For this review, take the finished solid that the model builds, in its own axes (mm). Give positions to 0.01 mm unless a question says otherwise; leave off trailing zeros. Order: outer loops, then holes, each group sorted by start corner. A loop starts at its lowest first (then second) coordinate and runs counter-clockwise, first axis right, second up. Notation, with made-up numbers: (43, -29.5) - (51, -29.5) arc R23 cw to (51, -8.5) - close; hole circle Ø11 at (88, 55.5). An arc over 180 degrees is marked (long way). One line per item, written item: value.
```python
from build123d import *

# Parameters (mm, degrees)
BOX032_W     = 40
BOX032_H     = 17
BOX032_DEPTH = 40
BOX033_W     = 40
BOX033_H     = 17
BOX033_DEPTH = 40
BOX029_W     = 330
BOX029_H     = 20
BOX029_DEPTH = 40
BOX030_W     = 30
BOX030_H     = 330
BOX030_DEPTH = 40
BOX031_W     = 30
BOX031_H     = 330
BOX031_DEPTH = 40
BOX028_W     = 330
BOX028_H     = 20
BOX028_DEPTH = 40
BOX009_W     = 64.5
BOX009_H     = 12
BOX009_DEPTH = 3
BOX008_W     = 64.5
BOX008_H     = 10
BOX008_DEPTH = 3
BOX007_W     = 22
BOX007_H     = 6
BOX007_DEPTH = 3
BOX006_W     = 22
BOX006_H     = 6
BOX006_DEPTH = 3
BOX005_W     = 22
BOX005_H     = 6
BOX005_DEPTH = 3
BOX004_W     = 74.5
BOX004_H     = 117
BOX004_DEPTH = 10
BOX003_W     = 74.5
BOX003_H     = 117
BOX003_DEPTH = 10
BOX002_W     = 74.5
BOX002_H     = 117
BOX002_DEPTH = 10
BOX_W        = 310
BOX_H        = 310
BOX_DEPTH    = 3
BOX010_W     = 64.5
BOX010_H     = 12
BOX010_DEPTH = 3


with BuildPart() as cube031:
    # Box032 → Box032 (new body)
    with BuildSketch(Plane(origin=(-20, 140, 0), x_dir=(1, 0, 0), z_dir=(0, 0, 1))):
        with Locations((20, 8.5)):
            Rectangle(BOX032_W, BOX032_H)
    extrude(amount=BOX032_DEPTH)


with BuildPart() as fusion001010002020:
    # Box033 → Box033 (new body)
    with BuildSketch(Plane(origin=(-20, -156, 0), x_dir=(1, 0, 0), z_dir=(0, 0, 1))):
        with Locations((20, 8.5)):
            Rectangle(BOX033_W, BOX033_H)
    extrude(amount=BOX033_DEPTH)

    # Fusion001010002020: union Cube031
    add(cube031.part)


with BuildPart() as cube028:
    # Box029 → Box029 (new body)
    with BuildSketch(Plane(origin=(-165, -159, 0), x_dir=(1, 0, 0), z_dir=(0, 0, 1))):
        with Locations((165, 10)):
            Rectangle(BOX029_W, BOX029_H)
    extrude(amount=BOX029_DEPTH)


with BuildPart() as cube029:
    # Box030 → Box030 (new body)
    with BuildSketch(Plane(origin=(-170, -170, 0), x_dir=(1, 0, 0), z_dir=(0, 0, 1))):
        with Locations((15, 165)):
            Rectangle(BOX030_W, BOX030_H)
    extrude(amount=BOX030_DEPTH)


with BuildPart() as cube030:
    # Box031 → Box031 (new body)
    with BuildSketch(Plane(origin=(140, -170, 0), x_dir=(1, 0, 0), z_dir=(0, 0, 1))):
        with Locations((15, 165)):
            Rectangle(BOX031_W, BOX031_H)
    extrude(amount=BOX031_DEPTH)


with BuildPart() as cut007:
    # Box028 → Box028 (new body)
    with BuildSketch(Plane(origin=(-165, 140, 0), x_dir=(1, 0, 0), z_dir=(0, 0, 1))):
        with Locations((165, 10)):
            Rectangle(BOX028_W, BOX028_H)
    extrude(amount=BOX028_DEPTH)

    # Fusion001010002021: union Cube028, Cube029, Cube030
    add(cube028.part)
    add(cube029.part)
    add(cube030.part)

    # Cut007: cut Fusion001010002020
    add(fusion001010002020.part, mode=Mode.SUBTRACT)


with BuildPart() as cube008:
    # Box009 → Box009 (new body)
    with BuildSketch(Plane(origin=(80.5, -72, 28), x_dir=(1, 0, 0), z_dir=(0, 0, 1))):
        with Locations((32.25, 6)):
            Rectangle(BOX009_W, BOX009_H)
    extrude(amount=BOX009_DEPTH)


with BuildPart() as cube007:
    # Box008 → Box008 (new body)
    with BuildSketch(Plane(origin=(-145, -155, 28), x_dir=(1, 0, 0), z_dir=(0, 0, 1))):
        with Locations((32.25, 5)):
            Rectangle(BOX008_W, BOX008_H)
    extrude(amount=BOX008_DEPTH)


with BuildPart() as cube006:
    # Box007 → Box007 (new body)
    with BuildSketch(Plane(origin=(-102.5, 124, 28), x_dir=(1, 0, 0), z_dir=(0, 0, 1))):
        with Locations((11, 3)):
            Rectangle(BOX007_W, BOX007_H)
    extrude(amount=BOX007_DEPTH)


with BuildPart() as cube005:
    # Box006 → Box006 (new body)
    with BuildSketch(Plane(origin=(80.5, 39, 28), x_dir=(1, 0, 0), z_dir=(0, 0, 1))):
        with Locations((11, 3)):
            Rectangle(BOX006_W, BOX006_H)
    extrude(amount=BOX006_DEPTH)


with BuildPart() as cube004:
    # Box005 → Box005 (new body)
    with BuildSketch(Plane(origin=(-102.5, -45, 28), x_dir=(1, 0, 0), z_dir=(0, 0, 1))):
        with Locations((11, 3)):
            Rectangle(BOX005_W, BOX005_H)
    extrude(amount=BOX005_DEPTH)


with BuildPart() as cube003:
    # Box004 → Box004 (new body)
    with BuildSketch(Plane(origin=(-155, 13, 24), x_dir=(1, 0, 0), z_dir=(0, 0, 1))):
        with Locations((37.25, 58.5)):
            Rectangle(BOX004_W, BOX004_H)
    extrude(amount=BOX004_DEPTH)


with BuildPart() as cube002:
    # Box003 → Box003 (new body)
    with BuildSketch(Plane(origin=(-155, -156, 24), x_dir=(1, 0, 0), z_dir=(0, 0, 1))):
        with Locations((37.25, 58.5)):
            Rectangle(BOX003_W, BOX003_H)
    extrude(amount=BOX003_DEPTH)


with BuildPart() as fusion:
    # Box002 → Box002 (new body)
    with BuildSketch(Plane(origin=(80.5, -72, 24), x_dir=(1, 0, 0), z_dir=(0, 0, 1))):
        with Locations((37.25, 58.5)):
            Rectangle(BOX002_W, BOX002_H)
    extrude(amount=BOX002_DEPTH)

    # Fusion: union Cube003, Cube002
    add(cube003.part)
    add(cube002.part)


with BuildPart() as cut:
    # Box → Box (new body)
    with BuildSketch(Plane(origin=(-155, -155, 28), x_dir=(1, 0, 0), z_dir=(0, 0, 1))):
        with Locations((155, 155)):
            Rectangle(BOX_W, BOX_H)
    extrude(amount=BOX_DEPTH)

    # Cut: cut Fusion
    add(fusion.part, mode=Mode.SUBTRACT)


with BuildPart() as cut008:
    # Box010 → Box010 (new body)
    with BuildSketch(Plane(origin=(-145, 13, 28), x_dir=(1, 0, 0), z_dir=(0, 0, 1))):
        with Locations((32.25, 6)):
            Rectangle(BOX010_W, BOX010_H)
    extrude(amount=BOX010_DEPTH)

    # Fusion001003: union Cube008, Cube007, Cube006, Cube005, Cube004, Cut
    add(cube008.part)
    add(cube007.part)
    add(cube006.part)
    add(cube005.part)
    add(cube004.part)
    add(cut.part)

    # Cut008: cut Cut007
    add(cut007.part, mode=Mode.SUBTRACT)


solid = cut008.part
```
(1) Wall thickness on line 1 (Y direction, x = 127.5, z = 30.6); line 2 (Y direction, x = 95, z = 28.75); line 3 (Y direction, x = -23.5, z = 28.7): over which ranges is each line inside the solid? List them lowest first. Write a range as from..to.
Answers below:
line 1: y = -139..-60, 45..140
line 2: y = -139..-60, 39..140
line 3: y = -139..140
(2) Take a section at C-C (y = 64). Write out the cut boundary in (x, z), then the cut area to 4 significant figures.
Answers below:
outline: (-80.5, 28) - (140, 28) - (140, 31) - (-80.5, 31) - close
area: 661.5 mm^2
(3) For P1, Ø1.5, axis at x = 82, z = 29.5, coming from the +Y side; P2, Ø0.9, axis at y = 43, z = 29, coming from the +X side; P3, Ø1.5, axis at y = 145.5, z = 30, coming from the -X side, all flat-tipped, find the tip position at first contact; note any pin that passes through.
Answers below:
P1: stops at y = 140
P2: stops at x = 102.5
P3: stops at x = -20
(4) Take a section at D-D (x = 30). Write out the cut boundary in (y, z), then the cut area to 3 significant figures.
Answers below:
outline: (-139, 28) - (140, 28) - (140, 31) - (-139, 31) - close
area: 837 mm^2
(5) Take a section at A-A (x = -95). Write out the cut boundary in (y, z).
Answers below:
outline: (-45, 28) - (25, 28) - (25, 31) - (-45, 31) - close; (124, 28) - (140, 28) - (140, 31) - (124, 31) - close
(6) Take a section at B-B (z = 28.9). Write out the cut boundary in (x, y), then the cut area to 3 significant figures.
Answers below:
outline: (-140, -39) - (-102.5, -39) - (-102.5, -45) - (-80.5, -45) - (-80.5, -139) - (-20, -139) - (-20, -155) - (20, -155) - (20, -139) - (140, -139) - (140, -60) - (80.5, -60) - (80.5, 39) - (102.5, 39) - (102.5, 45) - (140, 45) - (140, 140) - (20, 140) - (20, 155) - (-20, 155) - (-20, 140) - (-140, 140) - (-140, 130) - (-102.5, 130) - (-102.5, 124) - (-80.5, 124) - (-80.5, 25) - (-140, 25) - close
area: 61,300 mm^2
